from build123d import *

# Parameters (mm, degrees)
PARED_START                  = -36.1
SK_PARED_W                   = 100
SK_PARED_H                   = 95.3
PARED_DEPTH                  = 6.35
CABEZA_START                 = -36.1
SK_CABEZA_R                  = 50
CABEZA_DEPTH                 = 6.35
ASIENTO_1MM_START            = -29.75
SK_ASIENTO_1MM_R             = 42
SK_ASIENTO_1MM_R_2           = 29
ASIENTO_1MM_DEPTH            = 1
PASO_BOSS_J2_START           = -36.1
SK_PASO_BOSS_J2_R            = 29
PASO_BOSS_J2_DEPTH           = 7.35
PASANTES_M3_ESTATOR_J2_START = -36.1
SK_PASANTES_M3_ESTATOR_J2_R  = 1.7
PASANTES_M3_ESTATOR_J2_DEPTH = 7.35
SK_ROSCA_M3_DESDE_ABAJO_R    = 1.25
ROSCA_M3_DESDE_ABAJO_DEPTH   = 9


with BuildPart() as part:
    # Sk_Pared → Pared (new body)
    with BuildSketch(Plane(origin=(0, 0, 0), x_dir=(1, 0, 0), z_dir=(0, 1, 0)).offset(PARED_START)):
        with Locations((0, -124)):
            Rectangle(SK_PARED_W, SK_PARED_H)
    extrude(amount=PARED_DEPTH)

    # Sk_Cabeza → Cabeza (add)
    with BuildSketch(Plane(origin=(0, 0, 0), x_dir=(1, 0, 0), z_dir=(0, 1, 0)).offset(CABEZA_START)):
        with Locations((0, -170)):
            Circle(SK_CABEZA_R)
    extrude(amount=CABEZA_DEPTH)

    # Sk_Asiento_1mm → Asiento_1mm (add)
    with BuildSketch(Plane(origin=(0, 0, 0), x_dir=(1, 0, 0), z_dir=(0, 1, 0)).offset(ASIENTO_1MM_START)):
        with Locations(Location((0, -170, 0), (0, 0, 270))):
            Circle(SK_ASIENTO_1MM_R)
        with Locations(Location((0, -170, 0), (0, 0, 270))):
            Circle(SK_ASIENTO_1MM_R_2, mode=Mode.SUBTRACT)
    extrude(amount=ASIENTO_1MM_DEPTH)

    # Sk_Paso_boss_J2 → Paso_boss_J2 (cut)
    with BuildSketch(Plane(origin=(0, 0, 0), x_dir=(1, 0, 0), z_dir=(0, 1, 0)).offset(PASO_BOSS_J2_START)):
        with Locations(Location((0, -170, 0), (0, 0, 270))):
            Circle(SK_PASO_BOSS_J2_R)
    extrude(amount=PASO_BOSS_J2_DEPTH, mode=Mode.SUBTRACT)

    # Sk_Pasantes_M3_estator_J2 → Pasantes_M3_estator_J2 (cut)
    with BuildSketch(Plane(origin=(0, 0, 0), x_dir=(1, 0, 0), z_dir=(0, 1, 0)).offset(PASANTES_M3_ESTATOR_J2_START)):
        with Locations(Location((37, -170, 0), (0, 0, 270))):
            Circle(SK_PASANTES_M3_ESTATOR_J2_R)
        with Locations(Location((26.162950904, -196.162950904, 0), (0, 0, 270))):
            Circle(SK_PASANTES_M3_ESTATOR_J2_R)
        with Locations(Location((0, -207, 0), (0, 0, 270))):
            Circle(SK_PASANTES_M3_ESTATOR_J2_R)
        with Locations(Location((-26.162950904, -196.162950904, 0), (0, 0, 270))):
            Circle(SK_PASANTES_M3_ESTATOR_J2_R)
        with Locations(Location((-37, -170, 0), (0, 0, 270))):
            Circle(SK_PASANTES_M3_ESTATOR_J2_R)
        with Locations(Location((-26.162950904, -143.837049096, 0), (0, 0, 270))):
            Circle(SK_PASANTES_M3_ESTATOR_J2_R)
        with Locations(Location((0, -133, 0), (0, 0, 270))):
            Circle(SK_PASANTES_M3_ESTATOR_J2_R)
        with Locations(Location((26.162950904, -143.837049096, 0), (0, 0, 270))):
            Circle(SK_PASANTES_M3_ESTATOR_J2_R)
    extrude(amount=PASANTES_M3_ESTATOR_J2_DEPTH, mode=Mode.SUBTRACT)

    # Sk_Rosca_M3_desde_abajo → Rosca_M3_desde_abajo (cut)
    with BuildSketch(Plane(origin=(0, 0, 76.35), x_dir=(-1, 0, 0), z_dir=(0, 0, -1))):
        with Locations((42, -32.9225)):
            Circle(SK_ROSCA_M3_DESDE_ABAJO_R)
        with Locations((20, -32.9225)):
            Circle(SK_ROSCA_M3_DESDE_ABAJO_R)
        with Locations((-20, -32.9225)):
            Circle(SK_ROSCA_M3_DESDE_ABAJO_R)
        with Locations((-42, -32.9225)):
            Circle(SK_ROSCA_M3_DESDE_ABAJO_R)
    extrude(amount=-ROSCA_M3_DESDE_ABAJO_DEPTH, mode=Mode.SUBTRACT)


solid = part.part
Design review of the part built by this model. Coordinates are the model's own, in mm. A direction names the side the tool comes from. Coordinates: 2 decimals unless noted, no trailing zeros. Write each loop counter-clockwise with the first axis right and the second up, starting at its lowest first coordinate (ties: lowest second). Pieces come first, ordered by that corner, then holes. Notation, with made-up numbers: (-1.5, 30) - (54.5, 30) arc R28 ccw to (54.5, 53) - close; hole circle Ø6 at (33, 17.5). An arc over 180 degrees is marked (long way). One line per item, written item: value.
1) Add section C-C (x = -37). State the section outline as (y, z) points, plus the area to 3 significant figures.
Answer sheet:
outline: (-36.1, 76.35) - (-29.75, 76.35) - (-29.75, 150.13) - (-28.75, 150.13) - (-28.75, 168.3) - (-36.1, 168.3) - close; (-36.1, 171.7) - (-28.75, 171.7) - (-28.75, 189.87) - (-29.75, 189.87) - (-29.75, 203.63) - (-36.1, 203.63) - close
area: 823 mm2
2) Add section B-B (z = 133). State the section outline as (x, y) points.
Answer sheet:
outline: (-50, -36.1) - (-1.7, -36.1) - (-1.7, -28.75) - (-19.87, -28.75) - (-19.87, -29.75) - (-50, -29.75) - close; (1.7, -36.1) - (50, -36.1) - (50, -29.75) - (19.87, -29.75) - (19.87, -28.75) - (1.7, -28.75) - close
3) To check wall thickness, follow probe 1 along X at (y, z) = (-29.5, 170); probe 2 along Y at (x, z) = (20, 79.75); probe 3 along Z at (x, y) = (1.5, -34.5). State the ranges of each line that lie inside material, in increasing order.
Answer sheet:
probe 1: x = -42 to -38.7, -35.3 to -29, 29 to 35.3, 38.7 to 42
probe 2: y = -36.1 to -34.17, -31.67 to -29.75
probe 3: z = 76.35 to 132.2, 133.8 to 141.04, 198.96 to 206.2, 207.8 to 219.98
4) Add section D-D (z = 89). State the section outline as (x, y) points, plus the area to 3 significant figures.
Answer sheet:
outline: (-50, -36.1) - (50, -36.1) - (50, -29.75) - (-50, -29.75) - close
area: 635 mm2
5) Add section A-A (x = 0). State the section outline as (y, z) points, plus the area to 3 significant figures.
Answer sheet:
outline: (-36.1, 76.35) - (-29.75, 76.35) - (-29.75, 128) - (-28.75, 128) - (-28.75, 131.3) - (-36.1, 131.3) - close; (-36.1, 134.7) - (-28.75, 134.7) - (-28.75, 141) - (-36.1, 141) - close; (-36.1, 199) - (-28.75, 199) - (-28.75, 205.3) - (-36.1, 205.3) - close; (-36.1, 208.7) - (-28.75, 208.7) - (-28.75, 212) - (-29.75, 212) - (-29.75, 220) - (-36.1, 220) - close
area: 520 mm2
6) Mouldability with a two-part tool opening along X and no side actions: class faces 1 (the face through (-27.197, -32.476, 194.814)), 2 (the face through (50, -33, 125)), 3 (the face through (-1, -36.1, 131)) as +X half, -X half, draft (parallel to the pull), parting line (faces both ways), or undercut.
Answer sheet:
face 1: undercut
face 2: +X half
face 3: draft
7) For faces 4 (the face through (-50, -33, 125)), 5 (the face through (1.85, -29.26, 128.04)), list the 3-axis set-ups (+Z, -Z, +X, -X, +Y, -Y) from which the entire face can be reached by the end or side of a thin tool; tool diameter is ignored.
Answer sheet:
face 4: +Z, -Z, -X, +Y, -Y
face 5: +Y
8) Insertion check: pin 1 (1.2 mm diameter, centred on x = -20.5, y = -33, fed in from -Z); pin 2 (3 mm diameter, centred on x = 42, y = -32.92, fed in from +Z). Each pin has a flat end and moves straight along its axis. Give the tip position at first contact, or say it passes through.
Answer sheet:
pin 1: stops at z = 85.35
pin 2: stops at z = 199.32
